Here's how the part is built. I have some questions about the finished solid (model axes, mm). A direction names the side the tool comes from. Round coordinates to 2 decimals unless told otherwise and drop trailing zeros. Order: outer loops, then holes, each group sorted by start corner. A loop starts at its lowest first (then second) coordinate and runs counter-clockwise, first axis right, second up. Notation, with made-up numbers: (30.5, 88) -> (54.5, 88) arc R26 ccw to (54.5, 110) -> close; hole circle Ø3 at (32.25, 46.25). An arc over 180 degrees is marked (long way). Use a Markdown table: item, result. Add a question column.
from build123d import *

# Parameters (mm, degrees)
BOSS_EXTRUDE1_DEPTH = 10
SKETCH4_R           = 1.6
CUT_EXTRUDE2_DEPTH  = 7.75


with BuildPart() as part:
    # Sketch1 → Boss-Extrude1 (new body)
    with BuildSketch(Plane(origin=(0, 0, 0), x_dir=(1, 0, 0), z_dir=(0, 1, 0))):
        Polygon((6.25, 5), (6.25, 1.75), (13.75, 1.75), (13.75, -1.75), (6.25, -1.75), (6.25, -5), (-6.25, -5), (-6.25, 5), align=None)
    extrude(amount=BOSS_EXTRUDE1_DEPTH)

    # Sketch4 → Cut-Extrude2 (cut, through all)
    with BuildSketch(Plane.XY.offset(1.75)):
        with Locations((10.780263086, 5)):
            Circle(SKETCH4_R)
    extrude(amount=-CUT_EXTRUDE2_DEPTH, mode=Mode.SUBTRACT)


solid = part.part
(1) Please list where these lines run through material, in increasing order: probe 1 along X at (y, z) = (5, 2); probe 2 along Z at (x, y) = (6.75, 1.5); probe 3 along Y at (x, z) = (9.5, -1). Write a range as from..to.
(2) If we mould it in two halves opening along Y, with no side actions, what happens to faces 1 (the flat face through (2, 0, 0)), 2 (the cylindrical face through (9.51, 4.03, 0.02)), 3 (the flat face through (9, 5, -1.75))? For each: pulls with the +Y half, pulls with the -Y half, needs draft (parallel to the pull), parting line crosses it, or undercut.
(3) I want a section at D-D on y = 5. List the corners of the cut face in (x, z) for me.
(4) I want a section at C-C on x = 12. List the corners of the cut face in (y, z) for me, and give its area (3 significant figures).
(5) I want a section at B-B on z = -1. List the corners of the cut face in (x, y) for me.
(6) I'm going to push flat-ended pins straight in: P1, Ø3, axis at y = 3, z = 3.5, coming from the +X side; P2, Ø4, axis at x = 3.5, z = 2.5, coming from the -Y side. Where does each tip first touch, or does it pass through?
(7) I want a section at A-A on y = 2. List the corners of the cut face in (x, z) for me.
(8) On a 3-axis mill with a long thin cutter (end or side, diameter ignored), from which of +Z, -Z, +X, -X, +Y, -Y can I reach the whole of each face in a straight line? I mean faces 4 (the flat face through (6.25, 5, -3)), 5 (the flat face through (2, 10, 0)), 6 (the flat face through (6.25, 5, 3)). Say none if no direction works.
Output:
| question | item | result |
|---|---|---|
| 1 | probe 1 | -6.25..6.25 |
| 1 | probe 2 | -1.75..1.75 |
| 1 | probe 3 | 0..4.04, 5.96..10 |
| 2 | face 1 | pulls with the -Y half |
| 2 | face 2 | undercut |
| 2 | face 3 | needs draft |
| 3 | outline | (-6.25, -5) -> (6.25, -5) -> (6.25, -1.75) -> (9.18, -1.75) -> (9.18, 1.75) -> (6.25, 1.75) -> (6.25, 5) -> (-6.25, 5) -> close; (12.38, -1.75) -> (13.75, -1.75) -> (13.75, 1.75) -> (12.38, 1.75) -> close |
| 4 | outline | (0, -1.75) -> (3.96, -1.75) -> (3.96, 1.75) -> (0, 1.75) -> close; (6.04, -1.75) -> (10, -1.75) -> (10, 1.75) -> (6.04, 1.75) -> close |
| 4 | area | 27.8 mm² |
| 5 | outline | (-6.25, 0) -> (13.75, 0) -> (13.75, 10) -> (-6.25, 10) -> close; hole circle Ø3.2 at (10.78, 5) |
| 6 | P1 | x = 6.25 |
| 6 | P2 | y = 0 |
| 7 | outline | (-6.25, -5) -> (6.25, -5) -> (6.25, -1.75) -> (13.75, -1.75) -> (13.75, 1.75) -> (6.25, 1.75) -> (6.25, 5) -> (-6.25, 5) -> close |
| 8 | face 4 | -Z, +X, +Y, -Y |
| 8 | face 5 | +Z, -Z, +X, -X, +Y |
| 8 | face 6 | +Z, +X, +Y, -Y |
